Can you work these out from the model? Positions are in its coordinate system, mm. A direction names the side the tool comes from. Round coordinates to 2 decimals unless told otherwise and drop trailing zeros. Loops run counter-clockwise (first coordinate to the right, second up) from the corner with the lowest first, then second, coordinate; pieces in that order, holes last.
```python
from build123d import *

# Parameters (mm, degrees)
SKETCH2_W           = 46
SKETCH2_H           = 35.6
BOSS_EXTRUDE1_DEPTH = 32
CUT_EXTRUDE2_REACH  = 60.795
CUT_EXTRUDE3_REACH  = 51.55
SKETCH4_W           = 3
SKETCH4_H           = 1.5
FILLET1_R           = 4
FILLET2_R           = 8
FILLET3_R           = 0.6


with BuildPart() as part:
    # Sketch2 → Boss-Extrude1 (new body)
    with BuildSketch(Plane(origin=(0, 0, 0), x_dir=(1, 0, 0), z_dir=(0, 1, 0))):
        Rectangle(SKETCH2_W, SKETCH2_H)
    extrude(amount=BOSS_EXTRUDE1_DEPTH)

    # Sketch3 → Cut-Extrude2 (cut, up to next)
    with BuildSketch(Plane(origin=(23, 0, 0), x_dir=(0, 0, -1), z_dir=(1, 0, 0)), mode=Mode.PRIVATE) as cut_extrude2_sk1:
        with BuildLine():
            Line((-17.8, 25.6678015), (-16.849429134, 25.6678015))
            ThreePointArc((-16.849429134, 25.6678015), (0, 13.625659234), (16.849429134, 25.6678015))
            Line((16.849429134, 25.6678015), (17.8, 25.6678015))
            Line((17.8, 25.6678015), (17.8, 32))
            Line((17.8, 32), (-17.8, 32))
            Line((-17.8, 32), (-17.8, 25.6678015))
        make_face()
    cut_extrude2_tool1 = extrude(cut_extrude2_sk1.sketch, amount=-CUT_EXTRUDE2_REACH, mode=Mode.PRIVATE) & part.part
    add(cut_extrude2_tool1.solids().sort_by_distance((23, 24.200301, 0))[0], mode=Mode.SUBTRACT)

    # Sketch4 → Cut-Extrude3 (cut, up to next)
    with BuildSketch(Plane(origin=(0, 0, -17.8), x_dir=(-1, 0, 0), z_dir=(0, 0, -1)), mode=Mode.PRIVATE) as cut_extrude3_sk1:
        with Locations((-16.833333333, 9.6678015)):
            Rectangle(SKETCH4_W, SKETCH4_H)
    cut_extrude3_tool1 = extrude(cut_extrude3_sk1.sketch, amount=-CUT_EXTRUDE3_REACH, mode=Mode.PRIVATE) & part.part
    # Sketch4 → Cut-Extrude3 (cut, up to next)
    with BuildSketch(Plane(origin=(0, 0, -17.8), x_dir=(-1, 0, 0), z_dir=(0, 0, -1)), mode=Mode.PRIVATE) as cut_extrude3_sk2:
        with Locations((-7.666666667, 9.6678015)):
            Rectangle(SKETCH4_W, SKETCH4_H)
    cut_extrude3_tool2 = extrude(cut_extrude3_sk2.sketch, amount=-CUT_EXTRUDE3_REACH, mode=Mode.PRIVATE) & part.part
    # Sketch4 → Cut-Extrude3 (cut, up to next)
    with BuildSketch(Plane(origin=(0, 0, -17.8), x_dir=(-1, 0, 0), z_dir=(0, 0, -1)), mode=Mode.PRIVATE) as cut_extrude3_sk3:
        with Locations((7.666666667, 9.6678015)):
            Rectangle(SKETCH4_W, SKETCH4_H)
    cut_extrude3_tool3 = extrude(cut_extrude3_sk3.sketch, amount=-CUT_EXTRUDE3_REACH, mode=Mode.PRIVATE) & part.part
    # Sketch4 → Cut-Extrude3 (cut, up to next)
    with BuildSketch(Plane(origin=(0, 0, -17.8), x_dir=(-1, 0, 0), z_dir=(0, 0, -1)), mode=Mode.PRIVATE) as cut_extrude3_sk4:
        with Locations((16.833333333, 9.6678015)):
            Rectangle(SKETCH4_W, SKETCH4_H)
    cut_extrude3_tool4 = extrude(cut_extrude3_sk4.sketch, amount=-CUT_EXTRUDE3_REACH, mode=Mode.PRIVATE) & part.part
    add(cut_extrude3_tool1.solids().sort_by_distance((16.833333, 9.667801, -17.8))[0], mode=Mode.SUBTRACT)
    add(cut_extrude3_tool2.solids().sort_by_distance((7.666667, 9.667801, -17.8))[0], mode=Mode.SUBTRACT)
    add(cut_extrude3_tool3.solids().sort_by_distance((-7.666667, 9.667801, -17.8))[0], mode=Mode.SUBTRACT)
    add(cut_extrude3_tool4.solids().sort_by_distance((-16.833333, 9.667801, -17.8))[0], mode=Mode.SUBTRACT)

    # Fillet1
    fillet1_edges = [part.edges().sort_by_distance(p)[0] for p in [
        (16.833333333, 10.4178015, -17.8),
        (16.833333333, 10.4178015, 17.8),
        (7.666666667, 10.4178015, -17.8),
        (7.666666667, 10.4178015, 17.8),
        (-7.666666667, 10.4178015, -17.8),
        (-7.666666667, 10.4178015, 17.8),
        (-16.833333333, 10.4178015, -17.8),
        (-16.833333333, 10.4178015, 17.8),
    ]]
    fillet(fillet1_edges, radius=FILLET1_R)

    # Fillet2
    # the kernel refuses this fillet: 8 mm, written as the material it takes off along each edge
    with BuildSketch(Plane(origin=(32.455669225, 25.6678015, 17.8), x_dir=(0, -1, 0), z_dir=(-1, 0, 0))) as fillet2_piece_1:
        with BuildLine():
            CenterArc((3.78226769, -8), FILLET2_R, 90, 28.215129255)
            Line((0, -0.950570866), (-0.075645354, -0.809582283))
            ThreePointArc((-0.075645354, -0.809582283), (-0.16, -0.475285433), (-0.16, 0))
            Line((-0.16, 0), (0, 0.16))
            Line((0, 0.16), (3.78226769, 0.16))
            Line((3.78226769, 0.16), (3.78226769, 0))
        make_face()
    extrude(amount=64.91133845, mode=Mode.SUBTRACT)
    with BuildSketch(Plane(origin=(32.455669225, 25.6678015, -17.8), x_dir=(0, -1, 0), z_dir=(-1, 0, 0))) as fillet2_piece_2:
        with BuildLine():
            CenterArc((3.78226769, 8), FILLET2_R, 241.784870745, 28.215129255)
            Line((0, 0.950570866), (-0.075645354, 0.809582283))
            ThreePointArc((-0.075645354, 0.809582283), (-0.16, 0.475285433), (-0.16, 0))
            Line((-0.16, 0), (0, -0.16))
            Line((0, -0.16), (3.78226769, -0.16))
            Line((3.78226769, -0.16), (3.78226769, 0))
        make_face()
    extrude(amount=64.91133845, mode=Mode.SUBTRACT)

    # Fillet3
    fillet3_edges = [part.edges().sort_by_distance(p)[0] for p in [
        (0, 25.6678015, -16.849429134),
        (0, 25.6678015, 16.849429134),
    ]]
    fillet(fillet3_edges, radius=FILLET3_R)


solid = part.part
```
(1) If I drill on line 1 (X direction, y = 9.25, z = 4); line 2 (Y direction, x = -7, z = 14); line 3 (Y direction, x = -6.5, z = -2.5), over which ranges is the centre line in solid material (lowest first)?
(2) We'd pull the mould along X, two halves only. Please class faces 6 (the flat face through (0, 11, -17.8)), 7 (the flat face through (15.333, 10, 0)): released by +X, released by -X, zero draft, split by the parting line, or undercut.
(3) Suppose I cut it at B-B (y = 15). Write out the boundary of the cut face in (x, z).
(4) Which directions (+Z, -Z, +X, -X, +Y, -Y) give clear straight access to the entire face, cutting with the end or side of a thin tool? Please do faces 1 (the cylindrical face through (0.322, 23.095, -17.708)), 2 (the cylindrical face through (0.322, 23.062, 17.713)), 3 (the cylindrical face through (-7.69, 11.62, -16.66)), 4 (the cylindrical face through (7.69, 11.62, 16.66)), 5 (the flat face through (-17, 10.418, 0)).
(5) Suppose I cut it at C-C (z = -7.5). Write out the boundary of the cut face in (x, y), then the cut area to 3 significant figures.
(6) For pin 1 (3.5 mm diameter, centred on x = -8, z = 8, fed in from +Y); pin 2 (3.5 mm diameter, centred on x = 8, z = -5.5, fed in from +Y); pin 3 (0.9 mm diameter, centred on x = 16.5, z = 8.5, fed in from +Y), each with a flat end and sliding along its axis, tell me the tip position at first contact or that it passes through.
(7) Suppose I cut it at A-A (z = 0). Write out the boundary of the cut face in (x, y).
Check result:
1. line 1: x = -23 to -18.33, -15.33 to -9.17, -6.17 to 6.17, 9.17 to 15.33, 18.33 to 23
1. line 2: y = 0 to 8.92, 10.42 to 20.43
1. line 3: y = 0 to 8.92, 10.42 to 13.8
2. face 6: zero draft
2. face 7: undercut
3. outline: (-23, -17.8) - (23, -17.8) - (23, -6.86) - (-23, -6.86) - close; (-23, 6.86) - (23, 6.86) - (23, 17.8) - (-23, 17.8) - close
4. face 1: -Z, +X, -X, +Y
4. face 2: +Z, +X, -X, +Y
4. face 3: -Z
4. face 4: +Z
4. face 5: +Z, -Z
5. outline: (-23, 0) - (23, 0) - (23, 15.28) - (-23, 15.28) - close; hole (-18.33, 8.92) - (-15.33, 8.92) - (-15.33, 10.42) - (-18.33, 10.42) - close; hole (-9.17, 8.92) - (-6.17, 8.92) - (-6.17, 10.42) - (-9.17, 10.42) - close; hole (6.17, 8.92) - (9.17, 8.92) - (9.17, 10.42) - (6.17, 10.42) - close; hole (15.33, 8.92) - (18.33, 8.92) - (18.33, 10.42) - (15.33, 10.42) - close
5. area: 685 mm2
6. pin 1: stops at y = 16.53
6. pin 2: stops at y = 15.17
6. pin 3: stops at y = 16.04
7. outline: (-23, 0) - (23, 0) - (23, 13.63) - (-23, 13.63) - close; hole (-18.33, 8.92) - (-15.33, 8.92) - (-15.33, 10.42) - (-18.33, 10.42) - close; hole (-9.17, 8.92) - (-6.17, 8.92) - (-6.17, 10.42) - (-9.17, 10.42) - close; hole (6.17, 8.92) - (9.17, 8.92) - (9.17, 10.42) - (6.17, 10.42) - close; hole (15.33, 8.92) - (18.33, 8.92) - (18.33, 10.42) - (15.33, 10.42) - close
